Input: part model. Units: mm. Frame: model coordinates. A direction names the side the tool comes from. Give positions to 0.01 mm unless a question says otherwise; leave off trailing zeros. Loops run counter-clockwise (first coordinate to the right, second up) from the corner with the lowest first, then second, coordinate; pieces in that order, holes last. Notation, with made-up numbers: (8.25, 56) - (16.25, 56) arc R32 cw to (16.25, 92) - close; hole circle Ø2 at (-20, 31.5). An arc over 180 degrees is marked (long way). Answer as a JSON object with one key per item and string values.
from build123d import *

# Parameters (mm, degrees)
SKETCH1_R           = 2.25
BOSS_EXTRUDE1_DEPTH = 5


with BuildPart() as part:
    # Sketch1 → Boss-Extrude1 (new body)
    with BuildSketch(Plane(origin=(0, 0, 0), x_dir=(1, 0, 0), z_dir=(0, 1, 0))):
        Polygon((0, 55.733260811), (0, 12.733260811), (-65.613421019, 12.733260811), (-65.613421019, -54.266739189), (67.386578981, -54.266739189), (67.386578981, 55.733260811), align=None)
        with Locations((62.386578981, 40.733260811)):
            Circle(SKETCH1_R, mode=Mode.SUBTRACT)
        with Locations((62.386578981, 15.733260811)):
            Circle(SKETCH1_R, mode=Mode.SUBTRACT)
        with Locations((62.386578981, -9.266739189)):
            Circle(SKETCH1_R, mode=Mode.SUBTRACT)
        with Locations((62.386578981, -34.266739189)):
            Circle(SKETCH1_R, mode=Mode.SUBTRACT)
        with Locations((0.886578981, -49.266739189)):
            Circle(SKETCH1_R, mode=Mode.SUBTRACT)
        with Locations((-50.613421019, -49.266739189)):
            Circle(SKETCH1_R, mode=Mode.SUBTRACT)
        with Locations((52.386578981, -49.266739189)):
            Circle(SKETCH1_R, mode=Mode.SUBTRACT)
    extrude(amount=BOSS_EXTRUDE1_DEPTH)


solid = part.part
Item 1: Cut plane C-C (z = -27). Return loops of the section in (x, y), then the cut area to 3 significant figures.
Geometry check:
{"outline": "(0, 0) - (67.39, 0) - (67.39, 5) - (0, 5) - close", "area": "337 mm2"}
Item 2: Cut plane A-A (y = 2.9). Return loops of the section in (x, z), then the cut area to 3 significant figures.
Geometry check:
{"outline": "(-65.61, -12.73) - (0, -12.73) - (0, -55.73) - (67.39, -55.73) - (67.39, 54.27) - (-65.61, 54.27) - close; hole circle Ø4.5 at (-50.61, 49.27); hole circle Ø4.5 at (0.89, 49.27); hole circle Ø4.5 at (52.39, 49.27); hole circle Ø4.5 at (62.39, -40.73); hole circle Ø4.5 at (62.39, -15.73); hole circle Ø4.5 at (62.39, 9.27); hole circle Ø4.5 at (62.39, 34.27)", "area": "11,700 mm2"}
Item 3: Cut plane B-B (x = -33). Return loops of the section in (y, z), then the cut area to 3 significant figures.
Geometry check:
{"outline": "(0, -12.73) - (5, -12.73) - (5, 54.27) - (0, 54.27) - close", "area": "335 mm2"}
Item 4: Contact query for flat-ended pins moving along their axis: P1, Ø2.5, axis at x = -18, y = 2, coming from the -Z side; P2, Ø3.5, axis at x = 62.39, z = 34.27, coming from the +Y side. Output: stop coordinate, or through.
Geometry check:
{"P1": "stops at z = -12.73", "P2": "passes through"}
Item 5: Mould query, pull axis Z, two halves, no side actions, for faces 1 (the face through (63.425, 2.465, 11.263)), 2 (the face through (-32, 2, -12.733)), 3 (the face through (67.387, 2, 0)). Classes: released by +Z, released by -Z, zero draft, split by the parting line, or undercut.
Geometry check:
{"face 1": "undercut", "face 2": "released by -Z", "face 3": "zero draft"}
Item 6: Material intervals for line 1 (Z direction, x = 52, y = 3); line 2 (X direction, y = 0.8, z = -36); line 3 (X direction, y = 3.5, z = 8), sorted ascending. Write a range as [from, to].
Geometry check:
{"line 1": "z = [-55.73, 47.05], [51.48, 54.27]", "line 2": "x = [0, 67.39]", "line 3": "x = [-65.61, 60.53], [64.25, 67.39]"}
Item 7: Access query for faces 4 (the face through (0, 2, -35)), 5 (the face through (15, 0, 11)). Directions: +Z, -Z, +X, -X, +Y, -Y. A direction counts if a zero-diameter tool reaches every point of the face in a straight line with its end or side. Return the directions, or none.
Geometry check:
{"face 4": "-Z, -X, +Y, -Y", "face 5": "+Z, -Z, +X, -X, -Y"}
